Verification items for the finished model (mm, model axes). Round coordinates to 2 decimals unless told otherwise and drop trailing zeros. Order: outer loops, then holes, each group sorted by start corner. A loop starts at its lowest first (then second) coordinate and runs counter-clockwise, first axis right, second up.
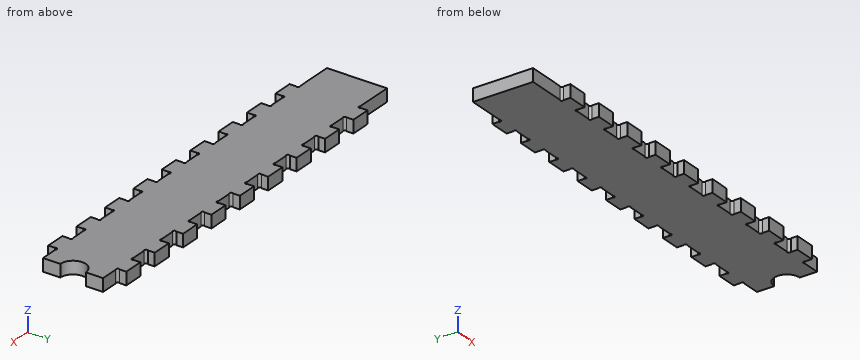
```python
from build123d import *

# Parameters (mm, degrees)
BOSS_EXTRUDE1_DEPTH = 6.35
SKETCH2_W           = 10.0254
SKETCH2_H           = 4.477133961
CUT_EXTRUDE2_DEPTH  = 204.051450213
LPATTERN1_COUNT     = 9
LPATTERN1_PITCH     = 20
CUT_EXTRUDE5_DEPTH  = 204.051450213


# Read off the part's stored shape, not the designer's step: Boss-Extrude1
with BuildPart() as part:
    # Boss-Extrude1 outline → Boss-Extrude1 (new body)
    with BuildSketch(Plane.XY):
        with BuildLine():
            Line((190, -4.490128061), (190, -1.122532015))
            ThreePointArc((190, -1.122532015), (190, 0), (191.122532015, 0))
            Line((191.122532015, 0), (200, 0))
            Line((200, 0), (200, 30))
            Line((200, 30), (191.122532015, 30))
            ThreePointArc((191.122532015, 30), (190, 30), (190, 31.122532015))
            Line((190, 31.122532015), (190, 34.490128061))
            Line((190, 34.490128061), (180, 34.490128061))
            Line((180, 34.490128061), (180, 31.122532015))
            ThreePointArc((180, 31.122532015), (180, 30), (178.877467985, 30))
            Line((178.877467985, 30), (171.122532015, 30))
            ThreePointArc((171.122532015, 30), (170, 30), (170, 31.122532015))
            Line((170, 31.122532015), (170, 34.490128061))
            Line((170, 34.490128061), (160, 34.490128061))
            Line((160, 34.490128061), (160, 31.122532015))
            ThreePointArc((160, 31.122532015), (160, 30), (158.877467985, 30))
            Line((158.877467985, 30), (151.122532015, 30))
            ThreePointArc((151.122532015, 30), (150, 30), (150, 31.122532015))
            Line((150, 31.122532015), (150, 34.490128061))
            Line((150, 34.490128061), (140, 34.490128061))
            Line((140, 34.490128061), (140, 31.122532015))
            ThreePointArc((140, 31.122532015), (140, 30), (138.877467985, 30))
            Line((138.877467985, 30), (131.122532015, 30))
            ThreePointArc((131.122532015, 30), (130, 30), (130, 31.122532015))
            Line((130, 31.122532015), (130, 34.490128061))
            Line((130, 34.490128061), (120, 34.490128061))
            Line((120, 34.490128061), (120, 31.122532015))
            ThreePointArc((120, 31.122532015), (120, 30), (118.877467985, 30))
            Line((118.877467985, 30), (111.122532015, 30))
            ThreePointArc((111.122532015, 30), (110, 30), (110, 31.122532015))
            Line((110, 31.122532015), (110, 34.490128061))
            Line((110, 34.490128061), (100, 34.490128061))
            Line((100, 34.490128061), (100, 31.122532015))
            ThreePointArc((100, 31.122532015), (100, 30), (98.877467985, 30))
            Line((98.877467985, 30), (91.122532015, 30))
            ThreePointArc((91.122532015, 30), (90, 30), (90, 31.122532015))
            Line((90, 31.122532015), (90, 34.490128061))
            Line((90, 34.490128061), (80, 34.490128061))
            Line((80, 34.490128061), (80, 31.122532015))
            ThreePointArc((80, 31.122532015), (80, 30), (78.877467985, 30))
            Line((78.877467985, 30), (71.122532015, 30))
            ThreePointArc((71.122532015, 30), (70, 30), (70, 31.122532015))
            Line((70, 31.122532015), (70, 34.490128061))
            Line((70, 34.490128061), (60, 34.490128061))
            Line((60, 34.490128061), (60, 31.122532015))
            ThreePointArc((60, 31.122532015), (60, 30), (58.877467985, 30))
            Line((58.877467985, 30), (51.122532015, 30))
            ThreePointArc((51.122532015, 30), (50, 30), (50, 31.122532015))
            Line((50, 31.122532015), (50, 34.490128061))
            Line((50, 34.490128061), (40, 34.490128061))
            Line((40, 34.490128061), (40, 31.122532015))
            ThreePointArc((40, 31.122532015), (40, 30), (38.877467985, 30))
            Line((38.877467985, 30), (31.122532015, 30))
            ThreePointArc((31.122532015, 30), (30, 30), (30, 31.122532015))
            Line((30, 31.122532015), (30, 34.490128061))
            Line((30, 34.490128061), (20, 34.490128061))
            Line((20, 34.490128061), (20, 31.122532015))
            ThreePointArc((20, 31.122532015), (20, 30), (18.877467985, 30))
            Line((18.877467985, 30), (0, 30))
            Line((0, 30), (0, 0))
            Line((0, 0), (18.877467985, 0))
            ThreePointArc((18.877467985, 0), (20, 0), (20, -1.122532015))
            Line((20, -1.122532015), (20, -4.490128061))
            Line((20, -4.490128061), (30, -4.490128061))
            Line((30, -4.490128061), (30, -1.122532015))
            ThreePointArc((30, -1.122532015), (30, 0), (31.122532015, 0))
            Line((31.122532015, 0), (38.877467985, 0))
            ThreePointArc((38.877467985, 0), (40, 0), (40, -1.122532015))
            Line((40, -1.122532015), (40, -4.490128061))
            Line((40, -4.490128061), (50, -4.490128061))
            Line((50, -4.490128061), (50, -1.122532015))
            ThreePointArc((50, -1.122532015), (50, 0), (51.122532015, 0))
            Line((51.122532015, 0), (58.877467985, 0))
            ThreePointArc((58.877467985, 0), (60, 0), (60, -1.122532015))
            Line((60, -1.122532015), (60, -4.490128061))
            Line((60, -4.490128061), (70, -4.490128061))
            Line((70, -4.490128061), (70, -1.122532015))
            ThreePointArc((70, -1.122532015), (70, 0), (71.122532015, 0))
            Line((71.122532015, 0), (78.877467985, 0))
            ThreePointArc((78.877467985, 0), (80, 0), (80, -1.122532015))
            Line((80, -1.122532015), (80, -4.490128061))
            Line((80, -4.490128061), (90, -4.490128061))
            Line((90, -4.490128061), (90, -1.122532015))
            ThreePointArc((90, -1.122532015), (90, 0), (91.122532015, 0))
            Line((91.122532015, 0), (98.877467985, 0))
            ThreePointArc((98.877467985, 0), (100, 0), (100, -1.122532015))
            Line((100, -1.122532015), (100, -4.490128061))
            Line((100, -4.490128061), (110, -4.490128061))
            Line((110, -4.490128061), (110, -1.122532015))
            ThreePointArc((110, -1.122532015), (110, 0), (111.122532015, 0))
            Line((111.122532015, 0), (118.877467985, 0))
            ThreePointArc((118.877467985, 0), (120, 0), (120, -1.122532015))
            Line((120, -1.122532015), (120, -4.490128061))
            Line((120, -4.490128061), (130, -4.490128061))
            Line((130, -4.490128061), (130, -1.122532015))
            ThreePointArc((130, -1.122532015), (130, 0), (131.122532015, 0))
            Line((131.122532015, 0), (138.877467985, 0))
            ThreePointArc((138.877467985, 0), (140, 0), (140, -1.122532015))
            Line((140, -1.122532015), (140, -4.490128061))
            Line((140, -4.490128061), (150, -4.490128061))
            Line((150, -4.490128061), (150, -1.122532015))
            ThreePointArc((150, -1.122532015), (150, 0), (151.122532015, 0))
            Line((151.122532015, 0), (158.877467985, 0))
            ThreePointArc((158.877467985, 0), (160, 0), (160, -1.122532015))
            Line((160, -1.122532015), (160, -4.490128061))
            Line((160, -4.490128061), (170, -4.490128061))
            Line((170, -4.490128061), (170, -1.122532015))
            ThreePointArc((170, -1.122532015), (170, 0), (171.122532015, 0))
            Line((171.122532015, 0), (178.877467985, 0))
            ThreePointArc((178.877467985, 0), (180, 0), (180, -1.122532015))
            Line((180, -1.122532015), (180, -4.490128061))
            Line((180, -4.490128061), (190, -4.490128061))
        make_face()
    extrude(amount=BOSS_EXTRUDE1_DEPTH)

    # Sketch2 → Cut-Extrude2 (cut, through all)
    with BuildSketch(Plane(origin=(0, 0, 0), x_dir=(-1, 0, 0), z_dir=(0, 0, -1))):
        with Locations((-35, 32.25156108)):
            Rectangle(SKETCH2_W, SKETCH2_H)
        with Locations((-35, -2.251561081)):
            Rectangle(SKETCH2_W, SKETCH2_H)
    cut_extrude2 = extrude(amount=-CUT_EXTRUDE2_DEPTH, mode=Mode.SUBTRACT)

    # LPattern1: Cut-Extrude2 ×9
    with Locations(*[(i * LPATTERN1_PITCH, 0, 0) for i in range(1, LPATTERN1_COUNT)]):
        add(cut_extrude2, mode=Mode.SUBTRACT)

    # Sketch6 → Cut-Extrude5 (cut, through all)
    with BuildSketch(Plane(origin=(0, 0, 0), x_dir=(-1, 0, 0), z_dir=(0, 0, -1))):
        with BuildLine():
            Line((-200, 8.65), (-200, 21.35))
            ThreePointArc((-200, 21.35), (-193.65, 15), (-200, 8.65))
        make_face()
    extrude(amount=-CUT_EXTRUDE5_DEPTH, mode=Mode.SUBTRACT)


solid = part.part
```
1) Sectioned sample at A-A on x = 54.5. Record the cut outline in (y, z), then the cut area to 4 significant figures.
2) Sectioned sample at B-B on y = 15. Record the cut outline in (x, z).
3) Scan lines: probe 1 along Y at (x, z) = (97, 1.5); probe 2 along X at (y, z) = (16.5, 3.5); probe 3 along X at (y, z) = (18, 1.25). Record each from-to range of solid material in increasing order.
4) Go/stop test with flat-tipped pins: pin 1 Ø2.5 at (y, z) = (-2.5, 2) entering from -X; pin 2 Ø1.9 at (x, z) = (174.5, 4) entering from -Y; pin 3 Ø2.5 at (y, z) = (-2.5, 3.5) entering from +X. Record where each tip stops, or that it passes through.
Returned:
1. outline: (0, 0) - (30, 0) - (30, 6.35) - (0, 6.35) - close
1. area: 190.5 mm2
2. outline: (0, 0) - (193.65, 0) - (193.65, 6.35) - (0, 6.35) - close
3. probe 1: y = 0 to 30
3. probe 2: x = 0 to 193.83
3. probe 3: x = 0 to 194.4
4. pin 1: stops at x = 20
4. pin 2: stops at y = 0
4. pin 3: stops at x = 189.99
